from build123d import *

# Parameters (mm, degrees)
CYLINDER084_R     = 2
CYLINDER084_DEPTH = 52
CYLINDER048_R     = 10
CYLINDER048_DEPTH = 8
CYLINDER049_R     = 12
CYLINDER049_DEPTH = 9


with BuildPart() as cylindre080:
    # Cylinder084 → Cylinder084 (new body)
    with BuildSketch(Plane(origin=(0, 19, -224), x_dir=(1, 0, 0), z_dir=(0, 0, 1))):
        Circle(CYLINDER084_R)
    extrude(amount=CYLINDER084_DEPTH)


with BuildPart() as obj1:
    # Cone → Cone (revolve)
    with BuildSketch(Plane(origin=(0, 18, -181), x_dir=(1, 0, 0), z_dir=(0, -1, 0))):
        Polygon((0, 0), (6, 0), (12, 10), (0, 10), align=None)
    revolve(axis=Axis((0, 18, -181), (0, 0, 1)))


with BuildPart() as cylindre044:
    # Cylinder048 → Cylinder048 (new body)
    with BuildSketch(Plane(origin=(0, 18, -170), x_dir=(1, 0, 0), z_dir=(0, 0, 1))):
        Circle(CYLINDER048_R)
    extrude(amount=CYLINDER048_DEPTH)


with BuildPart() as fusion046:
    # Cylinder049 → Cylinder049 (new body)
    with BuildSketch(Plane(origin=(0, 18, -171), x_dir=(1, 0, 0), z_dir=(0, 0, 1))):
        Circle(CYLINDER049_R)
    extrude(amount=CYLINDER049_DEPTH)

    # Cut036: cut Cylindre044
    add(cylindre044.part, mode=Mode.SUBTRACT)

    # Fusion024: union obj1
    add(obj1.part)

    # Fusion046: union Cylindre080
    add(cylindre080.part)


solid = fusion046.part
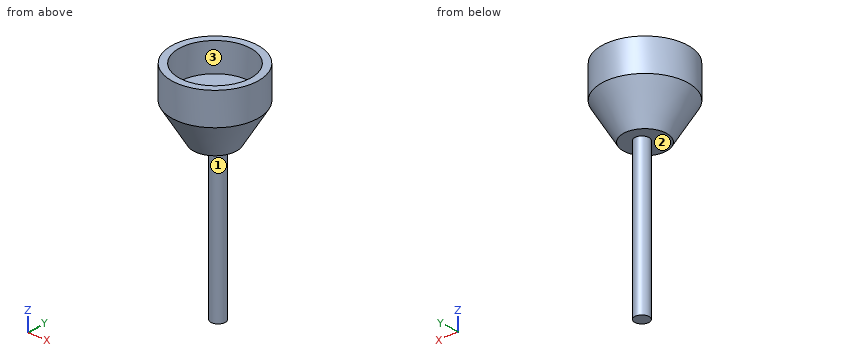
Design review of the part built by this model. Coordinates are the model's own, in mm. Face numbers are marked on the shaded views. Round coordinates to 2 decimals unless told otherwise and drop trailing zeros. Write each loop counter-clockwise with the first axis right and the second up, starting at its lowest first coordinate (ties: lowest second). Pieces come first, ordered by that corner, then holes. Notation, with made-up numbers: (44, 77.25) -> (90, 77.25) arc R8 cw to (90, 86.25) -> close; hole circle Ø7 at (65, -28.75). An arc over 180 degrees is marked (long way). One line per item, written item: value. Start each with the question number.
Q1. Add section B-B (y = 18). Give the boundary of the cut face in (x, z).
Q2. To check wall thickness, follow probe 1 along Y at (x, z) = (0, -166); probe 2 along Z at (x, y) = (5.25, 16); probe 3 along Y at (x, z) = (8.75, -166). State the ranges of each line that lie inside material, in increasing order.
Q3. The part is to be moulded in two halves that separate along Y. For the marked faces 1, 2 and 3, say which applies: pulls with the +Y half, pulls with the -Y half, needs draft (parallel to the pull), parting line crosses it, or undercut.
Q4. Add section D-D (z = -174.5). Give the boundary of the cut face in (x, y).
Q5. Add section C-C (z = -185). Give the boundary of the cut face in (x, y), then the cut area to 3 significant figures.
Q6. Insertion check: P1, Ø6, axis at x = 0.5, y = 16, coming from the -Z side; P2, Ø3, axis at x = -4, y = 17, coming from the +Z side; P3, Ø3, axis at x = 6, z = -183, coming from the +Y side; P4, Ø5, axis at y = 21.5, z = -186, coming from the -X side. Each pin has a flat end and moves straight along its axis. Give the tip position at first contact, or say it passes through.
Q7. Add section A-A (x = 0). Give the boundary of the cut face in (y, z), then the cut area to 3 significant figures.
Response:
1. outline: (-12, -171) -> (-6, -181) -> (-1.73, -181) -> (-1.73, -224) -> (1.73, -224) -> (1.73, -181) -> (6, -181) -> (12, -171) -> (12, -162) -> (10, -162) -> (10, -170) -> (-10, -170) -> (-10, -162) -> (-12, -162) -> close
2. probe 1: y = 6 to 8, 28 to 30
2. probe 2: z = -181 to -170
2. probe 3: y = 9.79 to 13.16, 22.84 to 26.21
3. face 1: parting line crosses it
3. face 2: needs draft
3. face 3: undercut
4. outline: circle Ø19.8 at (0, 18)
5. outline: circle Ø4 at (0, 19)
5. area: 12.6 mm^2
6. P1: stops at z = -224
6. P2: stops at z = -170
6. P3: passes through
6. P4: stops at x = -2
7. outline: (6, -171) -> (12, -181) -> (17, -181) -> (17, -224) -> (21, -224) -> (21, -181) -> (24, -181) -> (30, -171) -> (30, -162) -> (28, -162) -> (28, -170) -> (8, -170) -> (8, -162) -> (6, -162) -> close
7. area: 408 mm^2
